Verification items for the finished model (mm, model axes). A direction names the side the tool comes from. Give positions to 0.01 mm unless a question says otherwise; leave off trailing zeros. Order: outer loops, then holes, each group sorted by start corner. A loop starts at its lowest first (then second) coordinate and runs counter-clockwise, first axis right, second up. Notation, with made-up numbers: (-25.5, -25.5) - (9.5, -25.5) arc R16 cw to (9.5, 2.5) - close; hole circle Ø5 at (80, -7). An arc over 180 degrees is marked (long way). Answer as a JSON object with one key per item and string values. Group by question number.
(1) Depth check by flat-ended pin: pin 1 Ø3 at (x, y) = (14.5, 3.5) entering from -Z; pin 2 Ø5 at (x, y) = (-8, 6) entering from +Z; pin 3 Ø2 at (y, z) = (2.5, 4.5) entering from -X. Enter the tip coordinate at first touch or a pass-through.
(2) Access from +Z, -Z, +X, -X, +Y, -Y to the whole of each face (thin tool, end or side, straight path). Record for faces 5 (the face through (0, 10, -27)), 6 (the face through (-15.674, 5, -36)), 7 (the face through (-31.084, 4.93, -20.97)).
(3) Section check B-B (z = 4). Record the boundary of the cut face in (x, y), then the cut area to 3 significant figures.
(4) Mould release check, pull along Z, two halves, no side actions. Record for faces 1 (the face through (27.5, 4.9, -18.5)), 2 (the face through (13.156, 5, -38)), 3 (the face through (40.304, 4.93, -8.948)), 4 (the face through (-19.7, 4.9, -32.8)): +Z half, -Z half, draft (parallel to the pull), parting line (faces both ways), or undercut.
(5) Thickness scan on line 1 (X direction, y = 4, z = -38); line 2 (Z direction, x = 0, y = 2.75); line 3 (X direction, y = 2, z = -8). Record the ranges inside material, lowest first.
(6) Section check A-A (x = 0). Record the boundary of the cut face in (y, z).
```python
from build123d import *

# Parameters (mm, degrees)
BOSS_EXTRUDE1_DEPTH = 10


with BuildPart() as part:
    # Sketch1 → Boss-Extrude1 (new body)
    with BuildSketch(Plane(origin=(0, 0, 0), x_dir=(1, 0, 0), z_dir=(0, 1, 0))):
        with BuildLine():
            ThreePointArc((0, 30), (-13.892167355, 26.589616135), (-24.625826483, 17.133845746))
            ThreePointArc((-24.625826483, 17.133845746), (-28.62494362, 8.978452136), (-30, 0))
            ThreePointArc((-30, 0), (-26.261196487, -14.503432665), (-15.976696063, -25.391832996))
            ThreePointArc((-15.976696063, -25.391832996), (-12.874056383, -24.685697726), (-13.580191653, -21.583058047))
            ThreePointArc((-13.580191653, -21.583058047), (-12.327917765, 22.322017014), (25.5, 0))
            ThreePointArc((25.5, 0), (21.945347053, -12.986598583), (12.272412334, -22.352581406))
            ThreePointArc((12.272412334, -22.352581406), (13.029650018, -25.206692228), (15.976696063, -25.391832996))
            ThreePointArc((15.976696063, -25.391832996), (26.261196487, -14.503432665), (30, 0))
            ThreePointArc((30, 0), (28.624943418, 8.978452779), (24.625825713, 17.133846852))
            ThreePointArc((24.625825713, 17.133846852), (13.892166758, 26.589616447), (0, 30))
        make_face()
        with BuildLine():
            Line((-24.625826483, 17.133845746), (-33.577676267, 4.267691868))
            Line((-33.577676267, 4.267691868), (-30, 0))
            ThreePointArc((-30, 0), (-28.62494362, 8.978452136), (-24.625826483, 17.133845746))
        make_face()
        with BuildLine():
            Line((-36.964920826, 10.767390882), (-36.263797685, 10.279572292))
            Line((-36.263797685, 10.279572292), (-37.634960984, 8.308851333))
            ThreePointArc((-37.634960984, 8.308851333), (-38.27923419, 7.895694616), (-39.02695006, 8.059118652))
            Line((-39.02695006, 8.059118652), (-41.546608741, 9.812214895))
            ThreePointArc((-41.546608741, 9.812214895), (-41.959765459, 10.456488101), (-41.796341422, 11.204203971))
            Line((-41.796341422, 11.204203971), (-25.034897988, 35.294790347))
            ThreePointArc((-25.034897988, 35.294790347), (-24.390624781, 35.707947064), (-23.642908912, 35.544523027))
            Line((-23.642908912, 35.544523027), (-15.673976437, 30))
            Line((-15.673976437, 30), (-33.577676267, 4.267691868))
            Line((-33.577676267, 4.267691868), (-36.855117659, 6.548028579))
            ThreePointArc((-36.855117659, 6.548028579), (-37.268274376, 7.192301785), (-37.104850339, 7.940017655))
            Line((-37.104850339, 7.940017655), (-35.764584616, 9.866330702))
            Line((-35.764584616, 9.866330702), (-35.063461475, 9.378512113))
            ThreePointArc((-35.063461475, 9.378512113), (-34.315745606, 9.215088076), (-33.671472399, 9.628244793))
            Line((-33.671472399, 9.628244793), (-21.548947673, 27.051489405))
            ThreePointArc((-21.548947673, 27.051489405), (-21.385523636, 27.799205275), (-21.798680354, 28.443478482))
            Line((-21.798680354, 28.443478482), (-23.731037279, 29.787949338))
            ThreePointArc((-23.731037279, 29.787949338), (-24.478753149, 29.951373375), (-25.123026356, 29.538216658))
            Line((-25.123026356, 29.538216658), (-37.214653506, 12.159379958))
            ThreePointArc((-37.214653506, 12.159379958), (-37.378077543, 11.411664088), (-36.964920826, 10.767390882))
        make_face()
        with BuildLine():
            Line((-10.673976437, 33.521405271), (-10.673976437, 38.918895687))
            ThreePointArc((-10.673976437, 38.918895687), (-10.381083218, 39.626002468), (-9.673976437, 39.918895687))
            Line((-9.673976437, 39.918895687), (12.155554915, 39.918895687))
            ThreePointArc((12.155554915, 39.918895687), (12.862661696, 39.626002468), (13.155554915, 38.918895687))
            Line((13.155554915, 38.918895687), (13.155554915, 37.173234143))
            Line((13.155554915, 37.173234143), (15.673976437, 37.173234143))
            Line((15.673976437, 37.173234143), (15.673976437, 39.918895687))
            ThreePointArc((15.673976437, 39.918895687), (14.795296781, 42.040216031), (12.673976437, 42.918895687))
            Line((12.673976437, 42.918895687), (-14.673976437, 42.918895687))
            ThreePointArc((-14.673976437, 42.918895687), (-15.381083218, 42.626002468), (-15.673976437, 41.918895687))
            Line((-15.673976437, 41.918895687), (-15.673976437, 30))
            Line((-15.673976437, 30), (0, 30))
            Line((0, 30), (15.673976437, 30))
            Line((15.673976437, 30), (15.673976437, 35.267066815))
            Line((15.673976437, 35.267066815), (13.155554915, 35.267066815))
            Line((13.155554915, 35.267066815), (13.155554915, 33.521405271))
            ThreePointArc((13.155554915, 33.521405271), (12.862661696, 32.81429849), (12.155554915, 32.521405271))
            Line((12.155554915, 32.521405271), (-9.673976437, 32.521405271))
            ThreePointArc((-9.673976437, 32.521405271), (-10.381083218, 32.81429849), (-10.673976437, 33.521405271))
        make_face()
        with BuildLine():
            ThreePointArc((37.104850339, 7.940017655), (37.268274376, 7.192301785), (36.855117659, 6.548028579))
            Line((36.855117659, 6.548028579), (33.577676267, 4.267691868))
            Line((33.577676267, 4.267691868), (15.673976437, 30))
            Line((15.673976437, 30), (23.642908912, 35.544523027))
            ThreePointArc((23.642908912, 35.544523027), (24.390624781, 35.707947064), (25.034897988, 35.294790347))
            Line((25.034897988, 35.294790347), (41.796341422, 11.204203971))
            ThreePointArc((41.796341422, 11.204203971), (41.959765459, 10.456488101), (41.546608741, 9.812214895))
            Line((41.546608741, 9.812214895), (39.02695006, 8.059118652))
            ThreePointArc((39.02695006, 8.059118652), (38.27923419, 7.895694616), (37.634960984, 8.308851333))
            Line((37.634960984, 8.308851333), (36.263797685, 10.279572292))
            Line((36.263797685, 10.279572292), (36.964920826, 10.767390882))
            ThreePointArc((36.964920826, 10.767390882), (37.378077543, 11.411664088), (37.214653506, 12.159379958))
            Line((37.214653506, 12.159379958), (25.123026356, 29.538216658))
            ThreePointArc((25.123026356, 29.538216658), (24.478753149, 29.951373375), (23.731037279, 29.787949338))
            Line((23.731037279, 29.787949338), (21.798680354, 28.443478482))
            ThreePointArc((21.798680354, 28.443478482), (21.385523636, 27.799205275), (21.548947673, 27.051489405))
            Line((21.548947673, 27.051489405), (33.671472399, 9.628244793))
            ThreePointArc((33.671472399, 9.628244793), (34.315745606, 9.215088076), (35.063461475, 9.378512113))
            Line((35.063461475, 9.378512113), (35.764584616, 9.866330702))
            Line((35.764584616, 9.866330702), (37.104850339, 7.940017655))
        make_face()
        with BuildLine():
            Line((-15.673976437, 30), (-24.625826483, 17.133845746))
            ThreePointArc((-24.625826483, 17.133845746), (-13.892167355, 26.589616135), (0, 30))
            Line((0, 30), (-15.673976437, 30))
        make_face()
        with BuildLine():
            Line((15.673976437, 30), (0, 30))
            ThreePointArc((0, 30), (13.892166758, 26.589616447), (24.625825713, 17.133846852))
            Line((24.625825713, 17.133846852), (15.673976437, 30))
        make_face()
        with BuildLine():
            Line((33.577676267, 4.267691868), (24.625825713, 17.133846852))
            ThreePointArc((24.625825713, 17.133846852), (28.624943418, 8.978452779), (30, 0))
            Line((30, 0), (33.577676267, 4.267691868))
        make_face()
    extrude(amount=BOSS_EXTRUDE1_DEPTH)


solid = part.part
```
Solutions:
{
 "1": {"pin 1": "stops at z = -42.9", "pin 2": "stops at z = -23.24", "pin 3": "stops at x = -29.8"},
 "2": {"face 5": "+Z, -Z, +X, -X, +Y", "face 6": "-Z, +Y, -Y", "face 7": "+Y, -Y"},
 "3": {"outline": "(-29.73, 0) - (-25.18, 0) - (-25.18, 10) - (-29.73, 10) - close; (25.18, 0) - (29.73, 0) - (29.73, 10) - (25.18, 10) - close", "area": "91.0 mm2"},
 "4": {"face 1": "undercut", "face 2": "undercut", "face 3": "+Z half", "face 4": "-Z half"},
 "5": {"line 1": "x = -15.67 to -10.67, 13.16 to 15.67", "line 2": "z = -42.92 to -39.92, -32.52 to -25.5", "line 3": "x = -38.93 to -37.98, -37.06 to -24.21, 24.21 to 37.06, 37.98 to 38.93"},
 "6": {"outline": "(0, -42.92) - (10, -42.92) - (10, -39.92) - (0, -39.92) - close; (0, -32.52) - (10, -32.52) - (10, -25.5) - (0, -25.5) - close"}
}
